Here's the drawing with two shaded views (mm, measured from the low corner). I have some questions. Coordinates: 2 decimals unless noted, no trailing zeros.
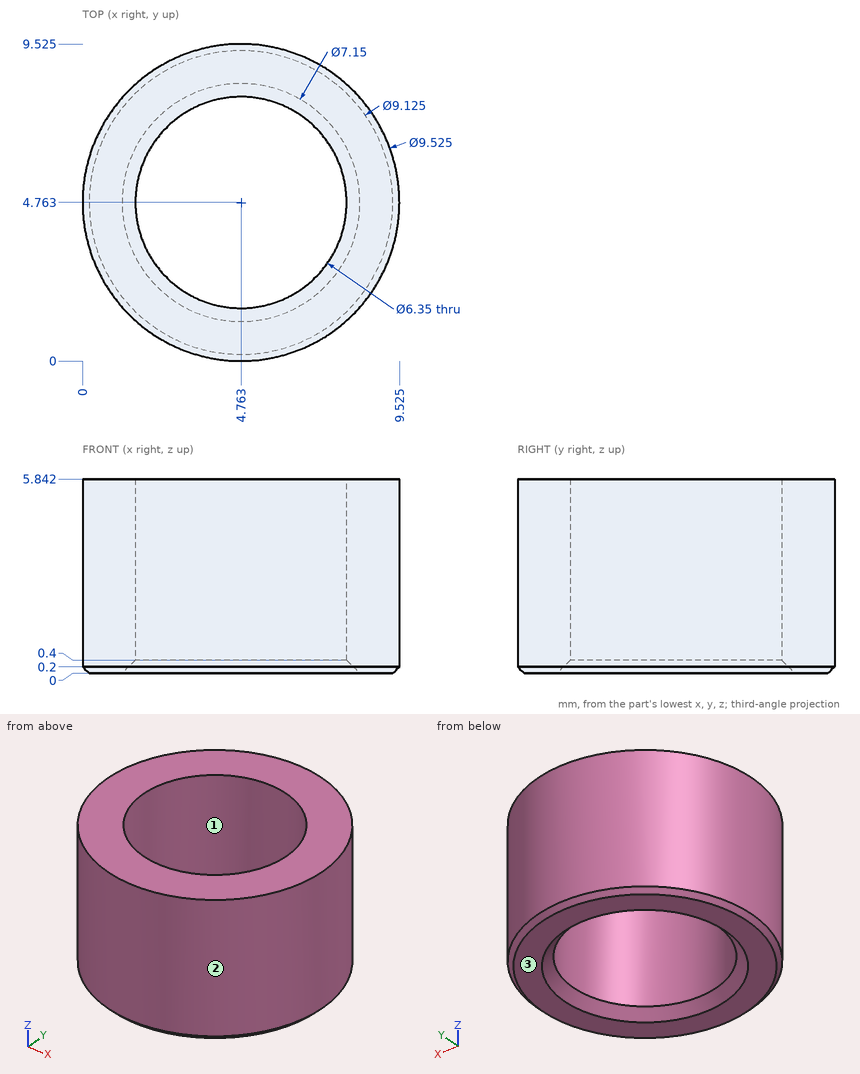
1. I'm going to push flat-ended pins straight in: P1, Ø1.5, axis at x = 4.5, y = 4, coming from the -Z side; P2, Ø1.5, axis at x = 1.5, z = 4.5, coming from the -Y side; P3, Ø2, axis at x = 6.5, z = 2.5, coming from the -Y side; P4, Ø1.5, axis at x = 2, y = 5, coming from the -Z side. Where does each tip first touch, or does it pass through?
2. We'd pull the mould along Y, two halves only. Please class the marked faces 1, 2 and 3: released by +Y, released by -Y, zero draft, split by the parting line, or undercut.
3. If I drill on L1, parallel to Y at x = 4.75, z = 4.1 (1 decimal); L2, parallel to Y at x = 6.5, z = 3.75 (1 decimal), over which ranges is the centre line in solid material (lowest first)?
Answers:
1. P1: passes through
1. P2: stops at y = 0.72
1. P3: stops at y = 0.06
1. P4: stops at z = 0.05
2. face 1: undercut
2. face 2: split by the parting line
2. face 3: zero draft
3. L1: y = 0 to 1.6, 7.9 to 9.5
3. L2: y = 0.3 to 2.1, 7.4 to 9.2
